from build123d import *

# Parameters (mm, degrees)
F0_R     = 6
F1_DEPTH = 20
F4_R     = 6
F4_R_2   = 2.75
F5_DEPTH = 15
F2_R     = 2.25
F6_DEPTH = 20
F8_DEPTH = 20
F9_SIZE  = 1


with BuildPart() as f1:
    # F0 (on Top) → F1 (new body)
    with BuildSketch(Plane.XY):
        Circle(F0_R)
    extrude(amount=-F1_DEPTH)

    # F4 (on offset) → F5 (join)
    with BuildSketch(Plane.XZ.offset(15)):
        with Locations((0, -10)):
            Circle(F4_R)
        with Locations((0, -10)):
            Circle(F4_R_2, mode=Mode.SUBTRACT)
    extrude(amount=-F5_DEPTH)

    # F2 (on face) → F6 (cut, through all)
    with BuildSketch(Plane.XY):
        Circle(F2_R)
    extrude(amount=-F6_DEPTH, mode=Mode.SUBTRACT)

    # F7 (on face) → F8 (cut, through all)
    with BuildSketch(Plane.XY):
        with BuildLine():
            Line((-1.0307764064, 2), (-5.6568542495, 2))
            ThreePointArc((-5.6568542495, 2), (-6, 0), (-5.6568542495, -2))
            Line((-5.6568542495, -2), (-1.0307764064, -2))
            ThreePointArc((-1.0307764064, -2), (-2.25, 0), (-1.0307764064, 2))
        make_face()
        with BuildLine():
            Line((0, 2), (-1.0307764064, 2))
            ThreePointArc((-1.0307764064, 2), (-2.25, 0), (-1.0307764064, -2))
            Line((-1.0307764064, -2), (0, -2))
            Line((0, -2), (0, 2))
        make_face()
        with BuildLine():
            Line((-5.6568542495, 2), (-8.5344118631, 2))
            Line((-8.5344118631, 2), (-8.5344118631, -2))
            Line((-8.5344118631, -2), (-5.6568542495, -2))
            ThreePointArc((-5.6568542495, -2), (-6, 0), (-5.6568542495, 2))
        make_face()
    extrude(amount=-F8_DEPTH, mode=Mode.SUBTRACT)

    # F9
    f9_edges = [f1.edges().sort_by_distance(p)[0] for p in [
        (-2.75, -15, -10),
    ]]
    chamfer(f9_edges, length=F9_SIZE)


solid = f1.part
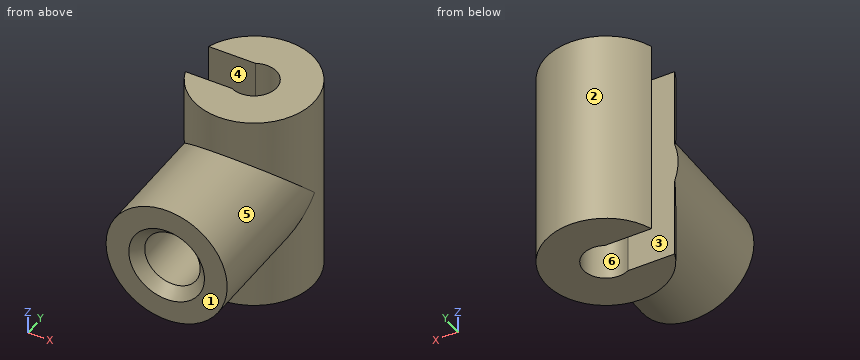
Source: CAD feature listing. Evaluate the final solid. Frame: model axes, mm. Face numbers are marked on the shaded views. A direction names the side the tool comes from. Round coordinates to 2 decimals unless told otherwise and drop trailing zeros. Order: outer loops, then holes, each group sorted by start corner. A loop starts at its lowest first (then second) coordinate and runs counter-clockwise, first axis right, second up. Notation, with made-up numbers: (73.5, 78.25) -> (98.5, 78.25) arc R34 ccw to (98.5, 109.25) -> close; hole circle Ø5 at (78, 84). An arc over 180 degrees is marked (long way). Answer as CSV lines item,"result".
Item 1: Reachability of the marked faces 4, 5 and 6 from +Z, -Z, +X, -X, +Y, -Y: full face, straight path, thin tool, end or side. Return the list, or none.
A:
face 4,"+Z, -Z, -X"
face 5,"-Y"
face 6,"+Z, -Z"
Item 2: Section C-C, the plane y = -4.75. Return loops of the section in (x, z), plus the area to 3 significant figures.
A:
outline,"(-3.67, -20) -> (3.67, -20) -> (3.67, -14.75) arc R6 ccw to (3.67, -5.25) -> (3.67, 0) -> (-3.67, 0) -> (-3.67, -5.25) arc R6 ccw to (-3.67, -14.75) -> close"
area,"178 mm²"
Item 3: Section A-A, the plane x = 0. Return loops of the section in (y, z).
A:
outline,"(-15, -16) -> (-6, -16) -> (-6, -20) -> (-2.25, -20) -> (-2.25, 0) -> (-6, 0) -> (-6, -4) -> (-15, -4) -> (-15, -6.25) -> (-14, -7.25) -> (-6, -7.25) -> (-6, -12.75) -> (-14, -12.75) -> (-15, -13.75) -> close; (2.25, -20) -> (6, -20) -> (6, 0) -> (2.25, 0) -> close"
Item 4: Pull-direction query (Y, two-part tool) for the marked faces 1, 2 and 3; classes: pulls with the +Y half, pulls with the -Y half, needs draft (parallel to the pull), parting line crosses it, or undercut.
A:
face 1,"pulls with the -Y half"
face 2,"parting line crosses it"
face 3,"undercut"
Item 5: Section D-D, the plane z = -5.5. Return loops of the section in (x, y), plus the area to 3 significant figures.
A:
outline,"(-5.66, -2) arc R6 ccw to (-3.97, -4.5) -> (-3.97, -15) -> (3.97, -15) -> (3.97, -4.5) arc R6 ccw (long way) to (-5.66, 2) -> (-1.03, 2) arc R2.25 cw (long way) to (-1.03, -2) -> close"
area,"156 mm²"
Item 6: Pin query (flat end, axial travel): pin 1 Ø1.5 at (x, z) = (-1, -15) entering from +Y; pin 2 Ø5.5 at (x, z) = (-4, -9.5) entering from +Y; pin 3 Ø1 at (y, z) = (-8, -4) entering from +X. Return the tip coordinate at first contact, or that it passes through.
A:
pin 1,"y = 5.99"
pin 2,"y = 5.87"
pin 3,"x = 2.4"
Item 7: Line query: L1, parallel to X at y = -8.75, z = -10; L2, parallel to Z at x = 0, y = -9; L3, parallel to Y at x = -2.5, z = -13. Output: solid intervals per line, ascending.
A:
L1,"-6 to -2.75, 2.75 to 6"
L2,"-16 to -12.75, -7.25 to -4"
L3,"-15 to -2, 2 to 5.45"
Item 8: Section B-B, the plane z = -10. Return loops of the section in (x, y), plus the area to 3 significant figures.
A:
outline,"(-6, -15) -> (-3.75, -15) -> (-2.75, -14) -> (-2.75, -5.33) arc R6 ccw to (2.75, -5.33) -> (2.75, -14) -> (3.75, -15) -> (6, -15) -> (6, 0) arc R6 ccw to (-5.66, 2) -> (-1.03, 2) arc R2.25 cw (long way) to (-1.03, -2) -> (-6, -2) -> close"
area,"153 mm²"
